```python
from build123d import *

# Parameters (mm, degrees)
SKETCH_1_W           = 99
SKETCH_1_H           = 65
EXTRUDE_1_DEPTH      = 2
EXTRUDE_2_DEPTH      = 46.5
EXTRUDE_2_DEPTH_BACK = 2
SKETCH_3_W           = 105
SKETCH_3_H           = 67
EXTRUDE_3_DEPTH      = 2
SKETCH_5_W           = 103
SKETCH_5_H           = 67
SKETCH_5_W_2         = 88
SKETCH_5_H_2         = 61
EXTRUDE_4_DEPTH      = 10
SKETCH_7_W           = 7
SKETCH_7_H           = 7
SKETCH_7_W_2         = 24.495718853
CUT_EXTRUDE_1_DEPTH  = 126.998015857
SKETCH_8_R           = 1.55
CUT_EXTRUDE_2_DEPTH  = 126.998015857
SKETCH_9_W           = 99.25
SKETCH_9_H           = 46.75
CUT_EXTRUDE_3_DEPTH  = 66
SKETCH_10_R          = 4
CUT_EXTRUDE_4_DEPTH  = 105.42940199
CUT_EXTRUDE_5_REACH  = 89.217
SKETCH_11_W          = 2
SKETCH_11_H          = 61.022672822
SKETCH_11_W_2        = 1
SKETCH_11_H_2        = 61


with BuildPart() as part:
    # 草图1 → 凸台-拉伸1 (new body)
    with BuildSketch(Plane(origin=(0, 0, 0), x_dir=(1, 0, 0), z_dir=(0, 1, 0))):
        Rectangle(SKETCH_1_W, SKETCH_1_H)
    extrude(amount=EXTRUDE_1_DEPTH)

    # 草图2 → 凸台-拉伸2 (add, two sides: drawn at the far end of the back side and taken through both)
    with BuildSketch(Plane(origin=(0, 2, 0), x_dir=(1, 0, 0), z_dir=(0, 1, 0)).offset(-EXTRUDE_2_DEPTH_BACK)):
        Polygon((-52.5, 34.5), (-52.5, -32.5), (-49.5, -32.5), (-49.5, 32.5), (49.5, 32.5), (49.5, -32.5), (52.5, -32.5), (52.5, 34.5), align=None)
    extrude(amount=EXTRUDE_2_DEPTH + EXTRUDE_2_DEPTH_BACK)

    # 草图3 → 凸台-拉伸3 (add)
    with BuildSketch(Plane(origin=(0, 48.5, 0), x_dir=(1, 0, 0), z_dir=(0, 1, 0))):
        with Locations((0, 1)):
            Rectangle(SKETCH_3_W, SKETCH_3_H)
    extrude(amount=EXTRUDE_3_DEPTH)

    # 草图5 → 凸台-拉伸4 (add)
    with BuildSketch(Plane(origin=(0, 50.5, 0), x_dir=(1, 0, 0), z_dir=(0, 1, 0))):
        with Locations((0.25, 1)):
            Rectangle(SKETCH_5_W, SKETCH_5_H)
        with Locations((0.25, 2)):
            Rectangle(SKETCH_5_W_2, SKETCH_5_H_2, mode=Mode.SUBTRACT)
    extrude(amount=EXTRUDE_4_DEPTH)

    # 草图7 → 切除-拉伸1 (cut, through all)
    with BuildSketch(Plane.ZY.offset(52.5)):
        with Locations((3, 41)):
            Rectangle(SKETCH_7_W, SKETCH_7_H)
        with Locations((25.747859426, 41)):
            Rectangle(SKETCH_7_W_2, SKETCH_7_H)
    extrude(amount=-CUT_EXTRUDE_1_DEPTH, mode=Mode.SUBTRACT)

    # 草图8 → 切除-拉伸2 (cut, through all)
    with BuildSketch(Plane.ZY.offset(52.5)):
        with Locations(Location((17.5, 53.5, 0), (0, 0, 180))):
            Circle(SKETCH_8_R)
        with Locations(Location((-2.5, 53.5, 0), (0, 0, 180))):
            Circle(SKETCH_8_R)
    extrude(amount=-CUT_EXTRUDE_2_DEPTH, mode=Mode.SUBTRACT)

    # 草图9 → 切除-拉伸3 (cut)
    with BuildSketch(Plane.XY.offset(32.5)):
        with Locations((0.125, 25.125)):
            Rectangle(SKETCH_9_W, SKETCH_9_H)
    extrude(amount=-CUT_EXTRUDE_3_DEPTH, mode=Mode.SUBTRACT)

    # 草图10 → 切除-拉伸4 (cut, through all)
    with BuildSketch(Plane.XY.offset(32.5)):
        with Locations((0, 21.301964842)):
            Circle(SKETCH_10_R)
    extrude(amount=-CUT_EXTRUDE_4_DEPTH, mode=Mode.SUBTRACT)

    # 草图11 → 切除-拉伸5 (cut, up to next)
    with BuildSketch(Plane(origin=(0, 60.5, 0), x_dir=(1, 0, 0), z_dir=(0, 1, 0)), mode=Mode.PRIVATE) as cut_extrude_5_sk1:
        with Locations((45.25, 1.988663589)):
            Rectangle(SKETCH_11_W, SKETCH_11_H)
    cut_extrude_5_tool1 = extrude(cut_extrude_5_sk1.sketch, amount=-CUT_EXTRUDE_5_REACH, mode=Mode.PRIVATE) & part.part
    # 草图11 → 切除-拉伸5 (cut, up to next)
    with BuildSketch(Plane(origin=(0, 60.5, 0), x_dir=(1, 0, 0), z_dir=(0, 1, 0)), mode=Mode.PRIVATE) as cut_extrude_5_sk2:
        with Locations((-44.25, 2)):
            Rectangle(SKETCH_11_W_2, SKETCH_11_H_2)
    cut_extrude_5_tool2 = extrude(cut_extrude_5_sk2.sketch, amount=-CUT_EXTRUDE_5_REACH, mode=Mode.PRIVATE) & part.part
    add(cut_extrude_5_tool1.solids().sort_by_distance((45.25, 60.5, -1.988664))[0], mode=Mode.SUBTRACT)
    add(cut_extrude_5_tool2.solids().sort_by_distance((-44.25, 60.5, -2))[0], mode=Mode.SUBTRACT)


solid = part.part
```
Could you check a few things on this model? Use its own coordinates, in mm. A direction names the side the tool comes from. Round coordinates to 2 decimals unless told otherwise and drop trailing zeros. Loops run counter-clockwise (first coordinate to the right, second up) from the corner with the lowest first, then second, coordinate; pieces in that order, holes last. Notation, with made-up numbers: M 67.25,6.5 L 97.25,6.5 A26 cw 97.25,37.5 Z; hole C 41.25,24.5 d3. An arc over 180 degrees is marked long. Put each result on its own line as item: value.
Q1. For pin 1 (1 mm diameter, centred on x = 16, z = -5, fed in from +Y); pin 2 (2 mm diameter, centred on x = 19.5, y = 40.5, fed in from +Z); pin 3 (11 mm diameter, centred on y = 57.5, z = 14, fed in from -X), each with a flat end and sliding along its axis, tell me the tip position at first contact or that it passes through.
Check result:
pin 1: y = 50.5
pin 2: z = -33.5
pin 3: x = -51.25
Q2. I need wall thicknesses on probe 1 along Y at (x, z) = (-46.25, 17.5); probe 2 along Z at (x, y) = (-47, 53.5); probe 3 along Y at (x, z) = (49.9, 17.5). Which ranges of each line are inside material? Lowest first, please.
Check result:
probe 1: 0 to 1.75, 48.5 to 51.95, 55.05 to 60.5
probe 2: -34.5 to -4.05, -0.95 to 15.95, 19.05 to 32.5
probe 3: 0 to 37.5, 44.5 to 51.95, 55.05 to 60.5
Q3. On a 3-axis mill with a long thin cutter (end or side, diameter ignored), from which of +Z, -Z, +X, -X, +Y, -Y can I reach the whole of each face in a straight line? I mean faces 1 (the face through (-51, 44.5, 23)), 2 (the face through (44.25, 50, -2)), 3 (the face through (-51, 41, 6.5)), 4 (the face through (-1, 1.75, 0)). Say none if no direction works.
Check result:
face 1: +Z, +X, -X
face 2: +Y
face 3: +X, -X
face 4: +Z
Q4. Imagine slicing it at D-D (z = -20). Write out the boundary of the cut face in (x, y), then the cut area to 3 significant figures.
Check result:
outline: M -52.5,0 L 52.5,0 L 52.5,50.5 L 51.75,50.5 L 51.75,60.5 L 46.25,60.5 L 46.25,48.5 L 49.75,48.5 L 49.75,1.75 L -49.5,1.75 L -49.5,48.5 L -44.75,48.5 L -44.75,60.5 L -51.25,60.5 L -51.25,50.5 L -52.5,50.5 Z; M -43.75,48.5 L 44.25,48.5 L 44.25,50.5 L -43.75,50.5 Z
area: 777 mm2
Q5. Imagine slicing it at A-A (z = -2.5). Write out the boundary of the cut face in (x, y), then the cut area to 3 significant figures.
Check result:
outline: M -52.5,0 L 52.5,0 L 52.5,50.5 L 51.75,50.5 L 51.75,51.95 L 46.25,51.95 L 46.25,48.5 L 49.75,48.5 L 49.75,1.75 L -49.5,1.75 L -49.5,48.5 L -44.75,48.5 L -44.75,51.95 L -51.25,51.95 L -51.25,50.5 L -52.5,50.5 Z; M -51.25,55.05 L -44.75,55.05 L -44.75,60.5 L -51.25,60.5 Z; M -43.75,48.5 L 44.25,48.5 L 44.25,50.5 L -43.75,50.5 Z; M 46.25,55.05 L 51.75,55.05 L 51.75,60.5 L 46.25,60.5 Z
area: 739 mm2
Q6. Thinking about a two-plate mould opening in X: for faces 5 (the face through (51.75, 55, -1)), 6 (the face through (1.846, 17.753, -33.993)), 7 (the face through (-1, 0, -1)), which applies, released by +X, released by -X, zero draft, split by the parting line, or undercut?
Check result:
face 5: released by +X
face 6: undercut
face 7: zero draft
Q7. Imagine slicing it at B-B (y = 53.5). State how many separate pieces and enclosed holes the cut face has, then the cut area to 3 significant figures.
Check result:
separate pieces: 4
enclosed holes: 0
area: 1,280 mm2
Q8. Imagine slicing it at C-C (x = 0). Write out the boundary of the cut face in (y, z).
Check result:
outline: M 0,-34.5 L 17.3,-34.5 L 17.3,-33.5 L 1.75,-33.5 L 1.75,32.5 L 0,32.5 Z; M 25.3,-34.5 L 60.5,-34.5 L 60.5,-32.5 L 50.5,-32.5 L 50.5,28.5 L 60.5,28.5 L 60.5,32.5 L 48.5,32.5 L 48.5,-33.5 L 25.3,-33.5 Z
